```python
from build123d import *

# Parameters (mm, degrees)
F1_DEPTH = 3
F3_DEPTH = 4.5


with BuildPart() as f1:
    # F0 (on Front) → F1 (new body, symmetric)
    with BuildSketch(Plane.XZ):
        with BuildLine():
            Line((0, 25), (0, 50))
            ThreePointArc((0, 50), (-12.5, 37.5), (0, 25))
        make_face()
        with BuildLine():
            ThreePointArc((0, 25), (8.838835, 28.661165), (12.5, 37.5))
            ThreePointArc((12.5, 37.5), (8.838835, 46.338835), (0, 50))
            Line((0, 50), (0, 25))
        make_face()
    extrude(amount=F1_DEPTH, both=True)

    # F2 (on Front) → F3 (join, symmetric)
    with BuildSketch(Plane.XZ):
        Polygon((6.5, 2.5), (0, 37.5), (-6.5, 2.5), align=None)
    extrude(amount=F3_DEPTH, both=True)

    # F4: F1 across plane


with BuildPart() as f1_1:
    add(f1.part)
    add(f1.part.mirror(Plane.XZ))


solid = f1_1.part
```
The listing builds one solid part. Answer for the finished solid, in the listing's coordinates (mm). A direction names the side the tool comes from. Coordinates: 2 decimals unless noted, no trailing zeros. Write each loop counter-clockwise with the first axis right and the second up, starting at its lowest first coordinate (ties: lowest second). Pieces come first, ordered by that corner, then holes. Notation, with made-up numbers: (7, -6) - (54, -6) arc R28 cw to (54, 19) - close; hole circle Ø3 at (55.5, 51.25). An arc over 180 degrees is marked (long way). Return JSON: item names as keys, results as strings. Group by question number.
1. Which of the six approach directions +Z, -Z, +X, -X, +Y, -Y give full straight-line access (tool end or side, diameter ignored) to faces 1 (the flat face through (0, 3, 38)), 2 (the flat face through (0, 4.5, 16))?
2. A cutting plane is placed at B-B, the plane z = 32. Determine the outline of the cut face in (x, y), plus the area to 3 significant figures.
3. Given pin 1 (8 mm diameter, centred on x = -8.5, z = 17.5, fed in from -Y); pin 2 (5 mm diameter, centred on y = -2, z = 21, fed in from +X), each flat-ended and moving along its own axis, determine where each tip first touches the part or whether it passes through.
4. Determine the mould class of faces 3 (the flat face through (0, -3, 38)), 4 (the flat face through (0, 0, 2.5)), 5 (the flat face through (-3.927, -0.063, 16.356)), 6 (the flat face through (4.018, -0.063, 15.866)) for opening direction Z: released by +Z, released by -Z, zero draft, split by the parting line, or undercut.
5. A cutting plane is placed at D-D, the plane x = 0.75. Determine the outline of the cut face in (y, z).
6. A cutting plane is placed at C-C, the plane y = -3.5. Determine the outline of the cut face in (x, z).
7. A cutting plane is placed at A-A, the plane x = -4.5. Determine the outline of the cut face in (y, z), plus the area to 3 significant figures.
8. Straight lines are drawn through the part: L1, parallel to Y at x = 8, z = 37; L2, parallel to X at y = 3, z = 20; L3, parallel to X at y = -2.75, z = 38. For each, find the intervals that lie inside material, in ascending order.
Ans:
{
 "1": {"face 1": "+Z, +Y", "face 2": "+Z, -Z, +X, -X, +Y"},
 "2": {"outline": "(-11.22, -3) - (-1.02, -3) - (-1.02, -4.5) - (1.02, -4.5) - (1.02, -3) - (11.22, -3) - (11.22, 3) - (1.02, 3) - (1.02, 4.5) - (-1.02, 4.5) - (-1.02, 3) - (-11.22, 3) - close", "area": "141 mm²"},
 "3": {"pin 1": "through", "pin 2": "x = 3.53"},
 "4": {"face 3": "zero draft", "face 4": "released by -Z", "face 5": "undercut", "face 6": "undercut"},
 "5": {"outline": "(-4.5, 2.5) - (4.5, 2.5) - (4.5, 33.46) - (3, 33.46) - (3, 49.98) - (-3, 49.98) - (-3, 33.46) - (-4.5, 33.46) - close"},
 "6": {"outline": "(-6.5, 2.5) - (6.5, 2.5) - (0, 37.5) - close"},
 "7": {"outline": "(-4.5, 2.5) - (4.5, 2.5) - (4.5, 13.27) - (-4.5, 13.27) - close; (-3, 25.84) - (3, 25.84) - (3, 49.16) - (-3, 49.16) - close", "area": "237 mm²"},
 "8": {"L1": "-3 to 3", "L2": "-3.25 to 3.25", "L3": "-12.49 to 12.49"}
}
